Read the model definition and answer for the solid it produces. Units are mm, in the model's axes. Face numbers are marked on the shaded views. A direction names the side the tool comes from. Coordinates: 2 decimals unless noted, no trailing zeros. Loops run counter-clockwise (first coordinate to the right, second up) from the corner with the lowest first, then second, coordinate; pieces in that order, holes last. Notation, with made-up numbers: M -1.5,85.25 L 4.5,85.25 A7 cw 4.5,92.25 Z; hole C -9,8.5 d4. An arc over 180 degrees is marked long. Put each result on its own line as item: value.
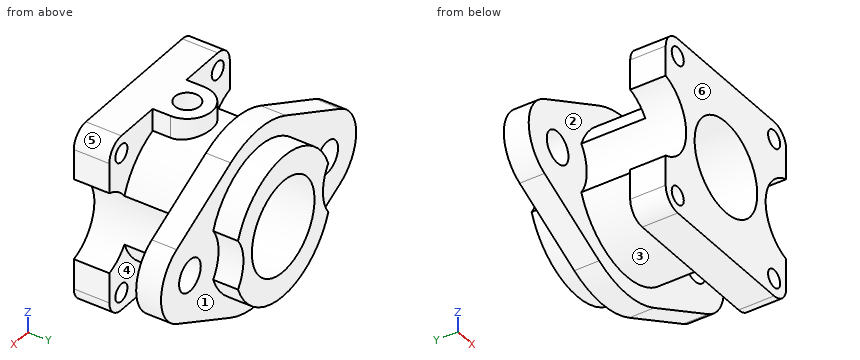
Autodesk Inventor part; units mm, degrees
ref_plane "Work Plane1" through (0, 28, 0) normal (0, -1, 0) x (1, 0, 0)
ref_plane "YZ Plane" through (0, 0, 0) normal (1, 0, 0) x (0, 1, 0)
ref_plane "XZ Plane" through (0, 0, 0) normal (0, 1, 0) x (-1, 0, 0)
sketch "Sketch1" plane through (0, 0, 0) normal (0, 1, 0) x (-1, 0, 0)
  line L0 (25, 25) -> (-25, 25)
  line L1 (-25, 25) -> (-25, -25)
  line L2 (-25, -25) -> (25, -25)
  line L3 (25, -25) -> (25, 25)
  line L4 (25, 25) -> (-25, -25) construction
  line L5 (-25, 25) -> (25, -25) construction
  point P0 (0, 0)
  dimension "d0" = 50
  dimension "d1" = 50
extrude "Extrusion1" add sketch "Sketch1" along normal blind 10
fillet "Fillet1" radius 5 4 edges at (-25, 5, -25) (-25, 5, 25) (25, 5, -25) (25, 5, 25)
sketch "Sketch2" plane through (0, 10, 0) normal (0, 1, 0) x (1, 0, 0)
  circle A0 centre (0, 0) radius 20
  dimension "d5" = 40
extrude "Extrusion2" add sketch "Sketch2" along normal blind 32
sketch "Sketch4" plane through (0, 0, 0) normal (0, -1, 0) x (1, 0, 0)
  circle A0 centre (-28.5, 0) radius 12
  line L0 (0, -36.4497) -> (0, 36.4497)
  circle A1 centre (28.5, 0) radius 12
  point P0 (0, 0)
  dimension "d14" = 12
  dimension "d15" = 57
extrude "Extrusion4" cut sketch "Sketch4" against normal through all
ref_plane "Work Plane1" through (0, 28, 0) normal (0, -1, 0) x (1, 0, 0)
sketch "Sketch3" plane through (0, 28, 0) normal (0, -1, 0) x (1, 0, 0)
  line L0 (-34.0605, -10.6894) -> (-11.3607, -22.2696)
  arc A0 (-11.3607, -22.2696) -> (11.4466, -22.2255) centre (0, 0) ccw
  line L1 (11.4466, -22.2255) -> (33.887, -10.6683)
  line L2 (33.887, -10.6683) -> (33.887, -10.6683)
  arc A1 (33.887, -10.6683) -> (33.887, 10.6683) centre (28.3926, 0) ccw
  line L3 (33.887, 10.6683) -> (11.4466, 22.2255)
  arc A2 (11.4466, 22.2255) -> (-11.3607, 22.2696) centre (0, 0) ccw
  arc A3 (-34.0605, 10.6894) -> (-34.0605, -10.6894) centre (-28.6074, 0) ccw
  line L4 (-11.3607, 22.2696) -> (-34.0605, 10.6894)
  dimension "d9" = 25
  dimension "d10" = 12
  dimension "d11" = 57
extrude "Extrusion3" add sketch "Sketch3" against normal blind 7
sketch "Sketch5" plane through (0, 42, 0) normal (0, 1, 0) x (1, 0, 0)
  arc A0 (18.7412, 6.9833) -> (-18.7412, 6.9833) centre (0, 0) ccw
hole "Hole1" at (0, 42, 0) direction (0, -1, 0) diameter 26 end through all
sketch "Sketch6" plane through (-20, 0, 25) normal (0, 0, 1) x (1, 0, 0)
  line L0 (0, 10) -> (40, 10)
  line L1 (0, 0) -> (40, 0)
  line L2 (1.2588, 10) -> (38.7412, 10)
  line L3 (13, 10) -> (13, 15)
  arc A0 (27, 15) -> (13, 15) centre (20, 15) ccw
  line L4 (27, 15) -> (27, 10)
  point P0 (20, 0)
  point P1 (20, 0)
  point P2 (20, 0)
  dimension "d25" = 7
  dimension "d26" = 15
extrude "Extrusion5" add sketch "Sketch6" against normal up to surface
sketch "Sketch7" plane through (-20, 0, 25) normal (0, 0, 1) x (1, 0, 0)
  arc A0 (27, 15) -> (13, 15) centre (20, 15) ccw
  point P0 (20, 0)
hole "Hole2" at (0, 15, 25) direction (0, 0, -1) diameter 7 end up to surface
sketch "Sketch8" plane through (0, 10, 0) normal (0, 1, 0) x (1, 0, 0)
  arc A0 (-25, -20) -> (-20, -25) centre (-20, -20) ccw
  arc A1 (25, 11.4782) -> (18.7412, 6.9833) centre (28.5, 0) ccw
  line L0 (25, 11.4782) -> (25, 20)
  arc A2 (25, 20) -> (20, 25) centre (20, 20) ccw
  line L1 (20, 25) -> (-20, 25)
  arc A3 (-20, 25) -> (-25, 20) centre (-20, 20) ccw
  line L2 (-25, 20) -> (-25, 11.4782)
  arc A4 (-18.7412, 6.9833) -> (-25, 11.4782) centre (-28.5, 0) ccw
  arc A5 (18.7412, 6.9833) -> (-18.7412, 6.9833) centre (0, 0) ccw
  line L3 (7, -18.735) -> (7, -25)
  line L4 (7, -25) -> (20, -25)
  arc A6 (20, -25) -> (25, -20) centre (20, -20) ccw
  line L5 (25, -20) -> (25, -11.4782)
  arc A7 (18.7412, -6.9833) -> (25, -11.4782) centre (28.5, 0) ccw
  arc A8 (7, -18.735) -> (18.7412, -6.9833) centre (0, 0) ccw
hole "Hole3" at (-20, 10, 20) at (20, 10, 20) at (-20, 10, -20) at (20, 10, -20) direction (0, -1, 0) diameter 5 end through all
sketch "Sketch9" plane through (0, 35, 0) normal (0, 1, 0) x (1, 0, 0)
  arc A0 (-34.0605, 10.6894) -> (-34.0605, -10.6894) centre (-28.6074, 0) ccw
  arc A1 (33.887, -10.6683) -> (33.887, 10.6683) centre (28.3926, 0) ccw
  point P0 (0, 0)
  point P1 (-28.6074, 0)
hole "Hole4" at (-28.6074, 35, 0) at (28.3926, 35, 0) direction (0, -1, 0) diameter 9 end through all
properties part number "Part025. Connection body" material "Steel, Carbon"
1) Which of the six approach directions +Z, -Z, +X, -X, +Y, -Y give full straight-line access (tool end or side, diameter ignored) to the marked faces 1, 2 and 3?
Answer list:
face 1: +Y
face 2: none
face 3: -Z
2) Find section A-A, the plane y = 5. Write down the section's boundary in (x, z), plus the area to 3 significant figures.
Answer list:
outline: M -25,-20 A5 ccw -20,-25 L 20,-25 A5 ccw 25,-20 L 25,-11.48 A12 cw 25,11.48 L 25,20 A5 ccw 20,25 L -20,25 A5 ccw -25,20 L -25,11.48 A12 cw -25,-11.48 Z; hole C -20,-20 d5; hole C -20,20 d5; hole C 0,0 d26; hole C 20,-20 d5; hole C 20,20 d5
area: 1,580 mm^2
3) Given pin 1 Ø12 at (y, z) = (29.5, -18.5) entering from +X; pin 2 Ø7 at (y, z) = (6, -17) entering from -X; pin 3 Ø4 at (y, z) = (11.5, 22.5) entering from +X, each flat-ended and moving along its own axis, determine where each tip first touches the part or whether it passes through.
Answer list:
pin 1: stops at x = 30.33
pin 2: stops at x = -25
pin 3: stops at x = 24.86
4) Straight lines are drawn through the part: line 1 (X direction, y = 2, z = -20); line 2 (Y direction, x = 15, z = 18.5); line 3 (X direction, y = 15, z = 20). For each, find the intervals that lie inside material, in ascending order. Write a range as [from, to].
Answer list:
line 1: x = [-25, -22.5], [-17.5, 17.5], [22.5, 25]
line 2: y = [0, 10], [28, 35]
line 3: x = [-7, -3.5], [3.5, 7]
5) Find section B-B, the plane x = 31. Write down the section's boundary in (y, z), plus the area to 3 significant figures.
Answer list:
outline: M 28,-12.16 L 35,-12.16 L 35,-3.67 L 28,-3.67 Z; M 28,3.67 L 35,3.67 L 35,12.16 L 28,12.16 Z
area: 119 mm^2
6) Find section C-C, the plane y = 37. Write down the section's boundary in (x, z).
Answer list:
outline: M -18.74,-6.98 A20 ccw 18.74,-6.98 A12 cw 18.74,6.98 A20 ccw -18.74,6.98 A12 cw Z; hole C 0,0 d26
7) Determine the mould class of the marked faces 4, 5 and 6 for opening direction Y: released by +Y, released by -Y, zero draft, split by the parting line, or undercut.
Answer list:
face 4: undercut
face 5: zero draft
face 6: released by -Y
